```python
from build123d import *

# Parameters (mm, degrees)
SKETCH2_R           = 5
BOSS_EXTRUDE1_DEPTH = 10
SKETCH3_R           = 4
CUT_EXTRUDE1_DEPTH  = 10


with BuildPart() as part:
    # Sketch2 → Boss-Extrude1 (new body)
    with BuildSketch(Plane.XY):
        with BuildLine():
            Line((-75, 90), (75, 90))
            ThreePointArc((75, 90), (85.606601718, 85.606601718), (90, 75))
            Line((90, 75), (90, -75))
            ThreePointArc((90, -75), (85.606601718, -85.606601718), (75, -90))
            Line((75, -90), (-75, -90))
            ThreePointArc((-75, -90), (-85.606601718, -85.606601718), (-90, -75))
            Line((-90, -75), (-90, 75))
            ThreePointArc((-90, 75), (-85.606601718, 85.606601718), (-75, 90))
        make_face()
        with Locations((-75, 75)):
            Circle(SKETCH2_R, mode=Mode.SUBTRACT)
        with Locations((0, 75)):
            Circle(SKETCH2_R, mode=Mode.SUBTRACT)
        with Locations((75, 75)):
            Circle(SKETCH2_R, mode=Mode.SUBTRACT)
        with Locations((-75, 0)):
            Circle(SKETCH2_R, mode=Mode.SUBTRACT)
        with Locations((75, 0)):
            Circle(SKETCH2_R, mode=Mode.SUBTRACT)
        with Locations((-75, -75)):
            Circle(SKETCH2_R, mode=Mode.SUBTRACT)
        with Locations((0, -75)):
            Circle(SKETCH2_R, mode=Mode.SUBTRACT)
        with Locations((75, -75)):
            Circle(SKETCH2_R, mode=Mode.SUBTRACT)
    extrude(amount=BOSS_EXTRUDE1_DEPTH)

    # Sketch3 → Cut-Extrude1 (cut)
    with BuildSketch(Plane.XY.offset(10)):
        Circle(SKETCH3_R)
    extrude(amount=-CUT_EXTRUDE1_DEPTH, mode=Mode.SUBTRACT)


solid = part.part
```
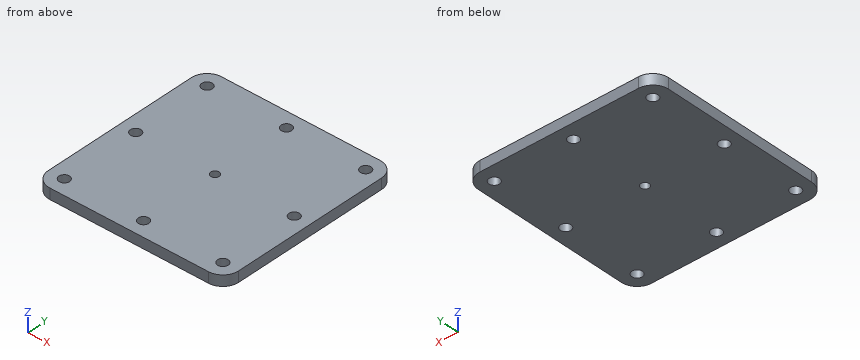
Work out the finished part from the listing and answer in its coordinate system (mm). Give positions to 0.01 mm unless a question says otherwise; leave off trailing zeros. Write each loop counter-clockwise with the first axis right and the second up, starting at its lowest first coordinate (ties: lowest second). Pieces come first, ordered by that corner, then holes. Notation, with made-up numbers: (-24, 47.5) -> (0, 47.5) arc R18 cw to (0, 59.5) -> close; hole circle Ø7 at (-1, 4). An arc over 180 degrees is marked (long way). Write each question's results on one line, items separated by ' | '.
1. Straight lines are drawn through the part: L1, parallel to Y at x = -75, z = 2.5; L2, parallel to Y at x = 0, z = 2.25; L3, parallel to X at y = 1, z = 0.5. For each, find the intervals that lie inside material, in ascending order.
Data:
L1: -90 to -80, -70 to -5, 5 to 70, 80 to 90 | L2: -90 to -80, -70 to -4, 4 to 70, 80 to 90 | L3: -90 to -79.9, -70.1 to -3.87, 3.87 to 70.1, 79.9 to 90
2. Find section B-B on z = 4. Give the number of separate pieces and of enclosed holes in the cut face, and give its area (3 significant figures).
Data:
separate pieces: 1 | enclosed holes: 9 | area: 31,500 mm^2
3. This flat-tipped pin is pushed along its axis until it touches: pin 1 Ø6 at (x, y) = (-75, 0) entering from -Z. Where does it stop, or does it pass through?
Data:
pin 1: through
4. Find section A-A on y = 0. Determine the outline of the cut face in (x, z), and give its area (3 significant figures).
Data:
outline: (-90, 0) -> (-80, 0) -> (-80, 10) -> (-90, 10) -> close; (-70, 0) -> (-4, 0) -> (-4, 10) -> (-70, 10) -> close; (4, 0) -> (70, 0) -> (70, 10) -> (4, 10) -> close; (80, 0) -> (90, 0) -> (90, 10) -> (80, 10) -> close | area: 1,520 mm^2
